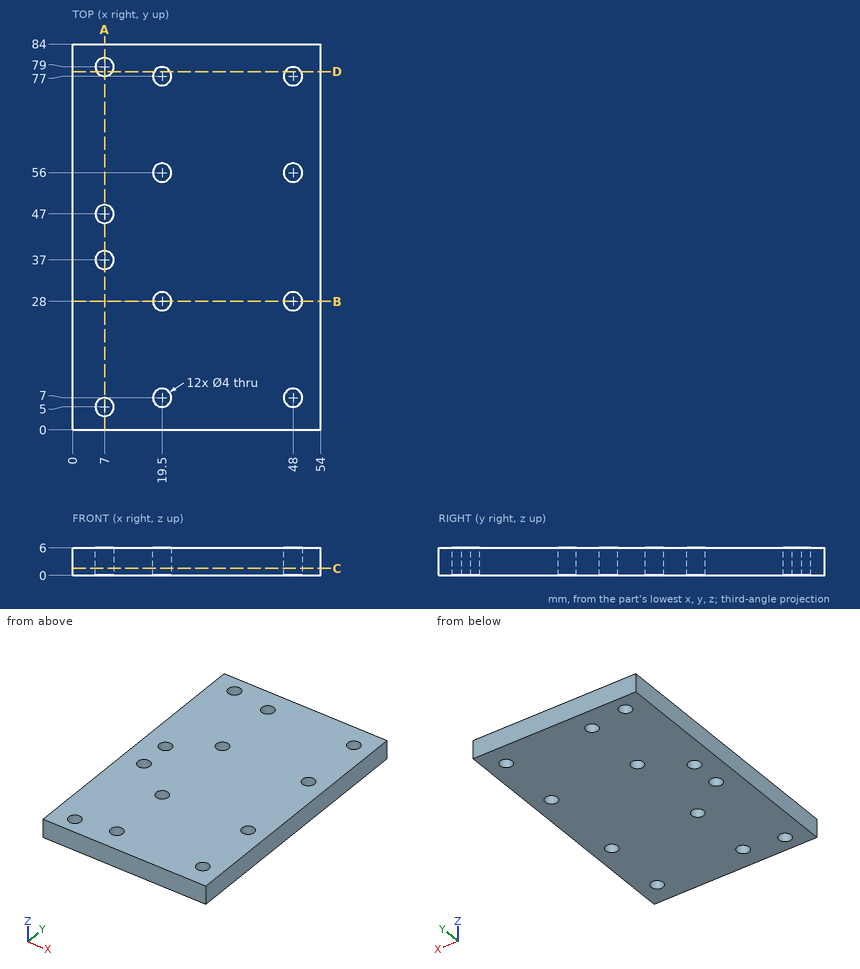
Study the drawing (mm; zero at the part's minimum x, y, z) and answer. Give positions to 0.01 mm unless a question says otherwise; leave off trailing zeros. Loops run counter-clockwise (first coordinate to the right, second up) from the corner with the lowest first, then second, coordinate; pieces in that order, holes last. Notation, with made-up numbers: (84, -2) -> (105, -2) arc R34 cw to (105, 30) -> close; hole circle Ø8 at (59, 15). An arc over 180 degrees is marked (long way). Use a Markdown table: item, result. Add a question column.
1) The part is cut by section C-C, the plane z = 1.55. Count the separate pieces of the cut face and the enclosed holes in it, plus the area to 3 significant figures.
2) This flat-tipped pin is pushed along its axis until it touches: P1, Ø2.5, axis at x = 48, y = 56, coming from the +Z side. Where does it stop, or does it pass through?
3) The part is cut by section D-D, the plane y = 78. Determine the outline of the cut face in (x, z).
4) The part is cut by section A-A, the plane x = 7. Determine the outline of the cut face in (y, z).
5) The part is cut by section B-B, the plane y = 28. Determine the outline of the cut face in (x, z).
6) Consider line 1 along X through (y, z) = (57, 0.9); line 2 along Y through (x, z) = (48, 2.6); line 3 along Y through (x, z) = (47.5, 2.55). Determine where each line is inside the solid, lowest interval first.
Reported:
| question | item | result |
|---|---|---|
| 1 | separate pieces | 1 |
| 1 | enclosed holes | 12 |
| 1 | area | 4,390 mm^2 |
| 2 | P1 | passes through |
| 3 | outline | (0, 0) -> (5.27, 0) -> (5.27, 6) -> (0, 6) -> close; (8.73, 0) -> (17.77, 0) -> (17.77, 6) -> (8.73, 6) -> close; (21.23, 0) -> (46.27, 0) -> (46.27, 6) -> (21.23, 6) -> close; (49.73, 0) -> (54, 0) -> (54, 6) -> (49.73, 6) -> close |
| 4 | outline | (0, 0) -> (3, 0) -> (3, 6) -> (0, 6) -> close; (7, 0) -> (35, 0) -> (35, 6) -> (7, 6) -> close; (39, 0) -> (45, 0) -> (45, 6) -> (39, 6) -> close; (49, 0) -> (77, 0) -> (77, 6) -> (49, 6) -> close; (81, 0) -> (84, 0) -> (84, 6) -> (81, 6) -> close |
| 5 | outline | (0, 0) -> (17.5, 0) -> (17.5, 6) -> (0, 6) -> close; (21.5, 0) -> (46, 0) -> (46, 6) -> (21.5, 6) -> close; (50, 0) -> (54, 0) -> (54, 6) -> (50, 6) -> close |
| 6 | line 1 | x = 0 to 17.77, 21.23 to 46.27, 49.73 to 54 |
| 6 | line 2 | y = 0 to 5, 9 to 26, 30 to 54, 58 to 75, 79 to 84 |
| 6 | line 3 | y = 0 to 5.06, 8.94 to 26.06, 29.94 to 54.06, 57.94 to 75.06, 78.94 to 84 |
